Geometry: final body of the model. Coordinates: model frame, mm. A direction names the side the tool comes from. Give positions to 0.01 mm unless a question says otherwise; leave off trailing zeros. Write each loop counter-clockwise with the first axis right and the second up, starting at its lowest first coordinate (ties: lowest second). Pieces come first, ordered by that corner, then holes. Notation, with made-up numbers: (-17, -33) - (20, -33) arc R34 cw to (20, -1) - close; hole circle Ø9 at (24.25, 34). An arc over 180 degrees is marked (long way). Use CSV: the item, a comma, the result in double quotes. Start each with the question number.
(1) Section C-C on x = 73. Output: boundary loops of the cut face in (y, z).
(2) First-contact query: pin 1 Ø1 at (x, y) = (59, -106) entering from -Z; pin 2 Ø4 at (x, z) = (60, 5) entering from -Y; pin 3 Ø4 at (x, z) = (60, 5) entering from +Y; pin 4 Ø2.5 at (x, y) = (6.5, -21.5) entering from +Z. Flat tips, straight axial feed; report the tip coordinate or a pass-through.
(3) Section B-B on y = -88.5. Output: boundary loops of the cut face in (x, z), and give its area (3 significant figures).
(4) Section A-A on x = 5. Output: boundary loops of the cut face in (y, z) (3 decimals).
(5) Draft query along Y for faces 1 (the conical face through (19.697, -136.908, 4.768)), 2 (the flat face through (9, -140, 8)), 3 (the cylindrical face through (7.218, -16.522, 6.549)). Return one class per face: released by +Y, released by -Y, zero draft, split by the parting line, or undercut.
(6) Line query: probe 1 along Z at (x, y) = (20, -9.25); probe 2 along X at (y, z) = (-20.5, 8); probe 3 along X at (y, z) = (-141.5, 5). Output: solid intervals per line, ascending. Write a range as [from, to].
(7) Reachability of faces 4 (the flat face through (5, -74, 10)), 5 (the cylindrical face through (4, -126, 7)), 6 (the cylindrical face through (62.1, -6.08, 5.66)), 7 (the cylindrical face through (3.817, -128.145, 1.479)), 8 (the flat face through (69, -74, 7)) from +Z, -Z, +X, -X, +Y, -Y: full face, straight path, thin tool, end or side. Return the list, or none.
from build123d import *

# Parameters (mm, degrees)
F1_DEPTH       = 150
F3_D           = 4.4
F3_DEPTH       = 12
F3_TIP         = 1.3218933619
F5_D           = 4.4
F5_DEPTH       = 12
F5_TIP         = 1.3218933619
F6_W           = 5
F6_H           = 3
F7_DEPTH       = 150
F9_D           = 4.4
F9_DEPTH       = 14.1
F9_START       = 3
F9_CBORE_D     = 8.25
F9_CBORE_DEPTH = 4
F9_TIP         = 1.3218933619


with BuildPart() as f1:
    # F0 (on Front) → F1 (new body)
    with BuildSketch(Plane.XZ):
        Polygon((0, 10), (0, 0), (70, 0), (80, 10), align=None)
    extrude(amount=F1_DEPTH)

    # F3
    with Locations(Plane.XZ.offset(150)):
        with Locations((20, 5), (60, 5)):
            Hole(F3_D / 2, depth=F3_DEPTH)
            with Locations((0, 0, -(F3_DEPTH + F3_TIP / 2))):  # 118° drill point
                Cone(0, F3_D / 2, F3_TIP, mode=Mode.SUBTRACT)

    # F5
    with Locations(Plane(origin=(0, 0, 0), x_dir=(-1, 0, 0), z_dir=(0, 1, 0))):
        with Locations((-60, 5), (-20, 5)):
            Hole(F5_D / 2, depth=F5_DEPTH)
            with Locations((0, 0, -(F5_DEPTH + F5_TIP / 2))):  # 118° drill point
                Cone(0, F5_D / 2, F5_TIP, mode=Mode.SUBTRACT)

    # F6 (on face) → F7 (cut, through all)
    with BuildSketch(Plane(origin=(0, 0, 0), x_dir=(-1, 0, 0), z_dir=(0, 1, 0))):
        with Locations((-68.5, 8.5)):
            Rectangle(F6_W, F6_H)
        with Locations((-11.5, 8.5)):
            Rectangle(F6_W, F6_H)
    extrude(amount=-F7_DEPTH, mode=Mode.SUBTRACT)

    # F9
    # its depths count from where the whole tool has entered the part; down to there all is cleared
    with Locations(Plane.XY.offset(10).offset(-F9_START)):
        with Locations((5, -130), (5, -20)):
            CounterBoreHole(F9_D / 2, F9_CBORE_D / 2, F9_CBORE_DEPTH, depth=F9_DEPTH)
            with Locations((0, 0, -(F9_DEPTH + F9_TIP / 2))):  # 118° drill point
                Cone(0, F9_D / 2, F9_TIP, mode=Mode.SUBTRACT)


solid = f1.part
Check values:
1,outline,"(-150, 3) - (0, 3) - (0, 10) - (-150, 10) - close"
2,pin 1,"stops at z = 0"
2,pin 2,"stops at y = -137.88"
2,pin 3,"stops at y = -12.12"
2,pin 4,"stops at z = 3"
3,outline,"(0, 0) - (70, 0) - (80, 10) - (71, 10) - (71, 7) - (66, 7) - (66, 10) - (14, 10) - (14, 7) - (9, 7) - (9, 10) - (0, 10) - close"
3,area,"720 mm²"
4,outline,"(-150, 0) - (-132.2, 0) - (-132.2, 3) - (-134.125, 3) - (-134.125, 10) - (-150, 10) - close; (-127.8, 0) - (-22.2, 0) - (-22.2, 3) - (-24.125, 3) - (-24.125, 10) - (-125.875, 10) - (-125.875, 3) - (-127.8, 3) - close; (-17.8, 0) - (0, 0) - (0, 10) - (-15.875, 10) - (-15.875, 3) - (-17.8, 3) - close"
5,face 1,"released by -Y"
5,face 2,"zero draft"
5,face 3,"undercut"
6,probe 1,"z = [0, 2.8], [7.2, 10]"
6,probe 2,"x = [0, 0.91], [14, 66], [71, 78]"
6,probe 3,"x = [0, 17.8], [22.2, 57.8], [62.2, 75]"
7,face 4,"+Z, +X, -X, +Y, -Y"
7,face 5,"+Z"
7,face 6,"+Y"
7,face 7,"+Z, -Z"
7,face 8,"+Z, +Y, -Y"
